Part model, mm, in its own coordinate system. A direction names the side the tool comes from. Coordinates: 2 decimals unless noted, no trailing zeros. Write each loop counter-clockwise with the first axis right and the second up, starting at its lowest first coordinate (ties: lowest second). Pieces come first, ordered by that corner, then holes. Notation, with made-up numbers: (8.5, 4.25) -> (19.5, 4.25) arc R32 ccw to (19.5, 31.25) -> close; hole circle Ø1 at (-9, 72.5). An arc over 180 degrees is marked (long way). Write item = value, one per line.
from build123d import *

# Parameters (mm, degrees)
SKETCH1_R           = 3.175
BOSS_EXTRUDE1_DEPTH = 54.5338
SKETCH2_R           = 2.667
BOSS_EXTRUDE2_DEPTH = 1.6002
SKETCH3_R           = 3.175
BOSS_EXTRUDE3_DEPTH = 2.286


with BuildPart() as part:
    # Sketch1 → Boss-Extrude1 (new body)
    with BuildSketch(Plane.XY):
        Circle(SKETCH1_R)
    extrude(amount=-BOSS_EXTRUDE1_DEPTH)

    # Sketch2 → Boss-Extrude2 (add)
    with BuildSketch(Plane.XY):
        Circle(SKETCH2_R)
    extrude(amount=BOSS_EXTRUDE2_DEPTH)

    # Sketch3 → Boss-Extrude3 (add)
    with BuildSketch(Plane.XY.offset(1.6002)):
        Circle(SKETCH3_R)
    extrude(amount=BOSS_EXTRUDE3_DEPTH)


solid = part.part
Q1. Saw through at A-A on y = 1.25. Give the cut face in (x, z), and give its area (3 significant figures).
Model answer:
outline = (-2.92, -54.53) -> (2.92, -54.53) -> (2.92, 0) -> (2.36, 0) -> (2.36, 1.6) -> (2.92, 1.6) -> (2.92, 3.89) -> (-2.92, 3.89) -> (-2.92, 1.6) -> (-2.36, 1.6) -> (-2.36, 0) -> (-2.92, 0) -> close
area = 339 mm²
Q2. Probe line 1 (Z direction, x = 1.5, y = 2.25); line 2 (Y direction, x = -0.25, z = -38); line 3 (Y direction, x = 2.75, z = -33). List the from-to ranges inside material, lowest first. Write a range as from..to.
Model answer:
line_1 = -54.53..0, 1.6..3.89
line_2 = -3.17..3.17
line_3 = -1.59..1.59
Q3. Saw through at C-C on z = -4.5. Give the cut face in (x, y) (3 decimals), and give its area (3 significant figures).
Model answer:
outline = circle Ø6.35 at (0, 0)
area = 31.7 mm²
Q4. Saw through at B-B on x = 0.75. Give the cut face in (y, z).
Model answer:
outline = (-3.09, -54.53) -> (3.09, -54.53) -> (3.09, 0) -> (2.56, 0) -> (2.56, 1.6) -> (3.09, 1.6) -> (3.09, 3.89) -> (-3.09, 3.89) -> (-3.09, 1.6) -> (-2.56, 1.6) -> (-2.56, 0) -> (-3.09, 0) -> close
Q5. Which spindle directions (+Z, -Z, +X, -X, +Y, -Y) get a long thin tool onto all of the face, cutting with end or side? Do faces 1 (the face through (-2, 2, 0)), 2 (the face through (0, 0, 3.886)). Say none if no direction does.
Model answer:
face_1 = none
face_2 = +Z, +X, -X, +Y, -Y
